Part model, mm, in its own coordinate system. A direction names the side the tool comes from. Round coordinates to 2 decimals unless told otherwise and drop trailing zeros. Loops run counter-clockwise (first coordinate to the right, second up) from the corner with the lowest first, then second, coordinate; pieces in that order, holes last. Notation, with made-up numbers: M 23,60 L 68,60 A15 cw 68,68 Z; hole C 61.5,78.5 d7. An arc over 180 degrees is marked long. Answer as CSV lines item,"result". Start each with the question number.
Item 1: Wall check: line 1 (Y direction, x = -1.5, z = -1.5); line 2 (X direction, y = -5.75, z = 0.5); line 3 (Y direction, x = -0.75, z = 0.75). Give the ranges that are in metal, low to high.
Item 2: Band-saw the part on D-D (y = 7.25). Give the cut face in (x, z) (1 decimal), and give its area (3 significant figures).
Item 3: Mould opens along Z. For faces 3 (the cylindrical face through (-0.31, 14.3, -1.39)), 4 (the cylindrical face through (-0.31, -5.4, 1.39)), 5 (the flat face through (0, 11.96, -2)) say: pulls with the +Z half, pulls with the -Z half, needs draft (parallel to the pull), parting line crosses it, or undercut.
Item 4: Band-saw the part on A-A (y = -5). Give the cut face in (x, z) (1 decimal), and give its area (3 significant figures).
Item 5: Which spindle directions (+Z, -Z, +X, -X, +Y, -Y) get a long thin tool onto all of the face, cutting with end or side? Do faces 1 (the flat face through (0, -2.273, 0)), 2 (the flat face through (-1.62, 1.81, 2.76)). Say none if no direction does.
Item 6: Band-saw the part on B-B (z = 0). Give the cut face in (x, y).
Item 7: Drop flat-ended pins along their axis: pin 1 Ø1.5 at (x, z) = (-2.5, 1) entering from +Y; pin 2 Ø1.5 at (x, y) = (0, 12.5) entering from +Z (3 decimals). Give the stop position or say it passes through.
Item 8: Band-saw the part on C-C (x = 0.5). Give the cut face in (y, z), and give its area (3 significant figures).
Autodesk Inventor part; units mm, degrees
ref_plane "YZ Plane" through (0, 0, 0) normal (1, 0, 0) x (0, 1, 0)
ref_plane "XZ Plane" through (0, 0, 0) normal (0, 1, 0) x (-1, 0, 0)
ref_plane "XY Plane" through (0, 0, 0) normal (0, 0, 1) x (1, 0, 0)
sketch "Sketch1" plane through (0, 0, 0) normal (0, 1, 0) x (-1, 0, 0)
  line L0 (3.2, 1.8475) -> (3.2, -1.8475)
  line L1 (3.2, -1.8475) -> (0, -3.695)
  line L2 (0, -3.695) -> (-3.2, -1.8475)
  line L3 (-3.2, -1.8475) -> (-3.2, 1.8475)
  line L4 (-3.2, 1.8475) -> (0, 3.695)
  line L5 (0, 3.695) -> (3.2, 1.8475)
  point P0 (0, 0)
  point P1 (3.2, 0)
  point P2 (-3.2, 0)
  dimension "d0" = 6.4
  dimension "d1" = 120
  dimension "d2" = 6.4
extrude "Extrusion1" add sketch "Sketch1" along normal blind 11.96
sketch "Sketch2" plane through (0, 11.96, 0) normal (0, 1, 0) x (1, 0, 0)
  circle A0 centre (0, 0) radius 1.4224
  dimension "d5" = 2.8448
extrude "Extrusion2" add sketch "Sketch2" along normal blind 4.75
sketch "Sketch3" plane through (0, 0, 0) normal (0, -1, 0) x (1, 0, 0)
  circle A0 centre (0, 0) radius 1.4224
  dimension "d8" = 2.8448
extrude "Extrusion3" cut sketch "Sketch3" against normal blind 6.35
sketch "Sketch4" plane through (0, 0, 0) normal (0, -1, 0) x (1, 0, 0)
  circle A0 centre (0, 0) radius 1.4224
  line L0 (-3.2, -1.8475) -> (-3.2, 1.8475)
  line L1 (0, -3.695) -> (-3.2, -1.8475)
  line L2 (3.2, -1.8475) -> (0, -3.695)
  line L3 (3.2, 1.8475) -> (3.2, -1.8475)
  line L4 (0, 3.695) -> (3.2, 1.8475)
  line L5 (-3.2, 1.8475) -> (0, 3.695)
extrude "Extrusion4" add sketch "Sketch4" along normal blind 8.6233
sketch "Sketch5" plane through (0, 6.35, 0) normal (0, -1, 0) x (1, 0, 0)
  circle A0 centre (0, 0) radius 1.4224
extrude "Extrusion5" add sketch "Sketch5" along normal blind 8.6233
properties part number "pc104standoffTEMP" material "Stainless Steel"
Answer block:
1,line 1,"y = -8.62 to 11.96"
1,line 2,"x = -3.2 to -1.33, 1.33 to 3.2"
1,line 3,"y = -2.27 to 16.71"
2,outline,"M -3.2,-1.8 L 0,-3.7 L 3.2,-1.8 L 3.2,1.8 L 0,3.7 L -3.2,1.8 Z"
2,area,"35.5 mm^2"
3,face 3,"parting line crosses it"
3,face 4,"undercut"
3,face 5,"needs draft"
4,outline,"M -3.2,-1.8 L 0,-3.7 L 3.2,-1.8 L 3.2,1.8 L 0,3.7 L -3.2,1.8 Z; hole C 0,0 d2.8"
4,area,"29.1 mm^2"
5,face 1,"-Y"
5,face 2,"+Z, -X, +Y, -Y"
6,outline,"M -3.2,-8.62 L -1.42,-8.62 L -1.42,-2.27 L 1.42,-2.27 L 1.42,-8.62 L 3.2,-8.62 L 3.2,11.96 L 1.42,11.96 L 1.42,16.71 L -1.42,16.71 L -1.42,11.96 L -3.2,11.96 Z"
7,pin 1,"stops at y = 11.96"
7,pin 2,"stops at z = 3.695"
8,outline,"M -8.62,-3.41 L 11.96,-3.41 L 11.96,-1.33 L 16.71,-1.33 L 16.71,1.33 L 11.96,1.33 L 11.96,3.41 L -8.62,3.41 L -8.62,1.33 L -2.27,1.33 L -2.27,-1.33 L -8.62,-1.33 Z"
8,area,"136 mm^2"
